Build history of the part. All positions in model axes, mm. Face numbers are marked on the shaded views. A direction names the side the tool comes from. Give positions to 0.01 mm unless a question says otherwise; leave off trailing zeros. Loops run counter-clockwise (first coordinate to the right, second up) from the corner with the lowest first, then second, coordinate; pieces in that order, holes last. Notation, with made-up numbers: (72, -26) -> (93, -26) arc R16 ccw to (93, -9) -> close; hole circle Ø4 at (18.25, 6). An arc over 180 degrees is marked (long way). Answer as a JSON object with one key per item and string values. Group by question number.
Q1. Band-saw the part on B-B, the plane x = 15. Write the cut outline in (y, z).
Q2. Tool access for the marked faces 4 and 5: list every direction of +Z, -Z, +X, -X, +Y, -Y with a clear straight run to the whole face (end or side of a thin tool).
Q3. Band-saw the part on A-A, the plane y = -3.75. Write the cut outline in (x, z).
Q4. Drop flat-ended pins along their axis: pin 1 (2 mm diameter, centred on y = -4, z = 7, fed in from +X); pin 2 (6 mm diameter, centred on x = 16.5, z = 12.5, fed in from -Y); pin 3 (2 mm diameter, centred on y = -3.5, z = 4.5, fed in from +X); pin 4 (2 mm diameter, centred on x = 13, y = -2.5, fed in from -Z). Give the stop position or say it passes through.
Q5. Band-saw the part on D-D, the plane z = 13.5. Write the cut outline in (x, y), plus the area to 3 significant figures.
Q6. Wall check: probe 1 along X at (y, z) = (-3.85, 11.75); probe 2 along X at (y, z) = (-1.45, 7.5); probe 3 along Z at (x, y) = (13.5, -1.4). Give the ranges that are in metal, low to high. Write a range as from..to.
Q7. Band-saw the part on C-C, the plane z = 7.5. Write the cut outline in (x, y).
Q8. Two-plate mould, pull along X, no slides. Class the marked faces 1, 2 and 3: pulls with the +X half, pulls with the -X half, needs draft (parallel to the pull), parting line crosses it, or undercut.
from build123d import *

# Parameters (mm, degrees)
BOSS_EXTRUDE1_DEPTH = 15
FILLET1_R           = 1
FILLET2_R           = 1
FILLET3_R           = 1
FILLET4_R           = 1
SKETCH2_R           = 2.25
CUT_EXTRUDE1_DEPTH  = 5


with BuildPart() as part:
    # Sketch1 → Boss-Extrude1 (new body)
    with BuildSketch(Plane.XY):
        Polygon((0, 0), (45, 0), (45, -2), (30, -2), (30, -5), (25, -5), (25, -2), (5, -2), (5, -5), (0, -5), align=None)
    extrude(amount=BOSS_EXTRUDE1_DEPTH)

    # Fillet1
    fillet1_edges = [part.edges().sort_by_distance(p)[0] for p in [
        (0, 0, 7.5),
    ]]
    fillet(fillet1_edges, radius=FILLET1_R)

    # Fillet2
    fillet2_edges = [part.edges().sort_by_distance(p)[0] for p in [
        (5, -2, 7.5),
    ]]
    fillet(fillet2_edges, radius=FILLET2_R)

    # Fillet3
    fillet3_edges = [part.edges().sort_by_distance(p)[0] for p in [
        (25, -2, 7.5),
    ]]
    fillet(fillet3_edges, radius=FILLET3_R)

    # Fillet4
    fillet4_edges = [part.edges().sort_by_distance(p)[0] for p in [
        (30, -2, 7.5),
    ]]
    fillet(fillet4_edges, radius=FILLET4_R)

    # Sketch2 → Cut-Extrude1 (cut)
    with BuildSketch(Plane(origin=(0, 0, 0), x_dir=(1, 0, 0), z_dir=(0, 1, 0))):
        with Locations(Location((15, -7.5, 0), (0, 0, 270))):
            Circle(SKETCH2_R)
    extrude(amount=-CUT_EXTRUDE1_DEPTH, mode=Mode.SUBTRACT)


solid = part.part
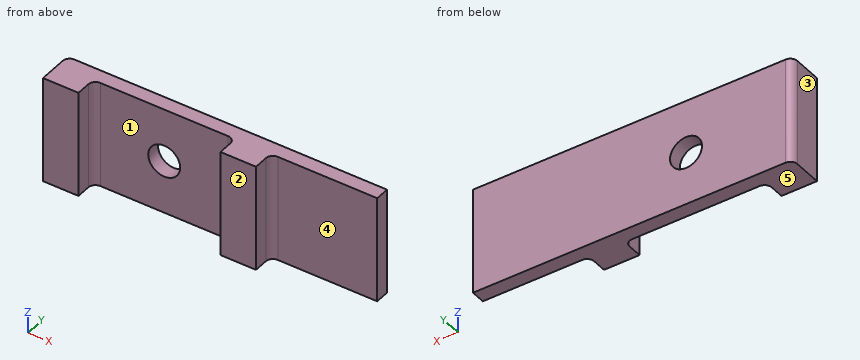
Worked answers:
{
 "1": {"outline": "(-2, 0) -> (0, 0) -> (0, 5.25) -> (-2, 5.25) -> close; (-2, 9.75) -> (0, 9.75) -> (0, 15) -> (-2, 15) -> close"},
 "2": {"face 4": "+Z, -Z, +X, -Y", "face 5": "-Z, +X, -X, +Y, -Y"},
 "3": {"outline": "(0, 0) -> (5, 0) -> (5, 15) -> (0, 15) -> close; (25, 0) -> (30, 0) -> (30, 15) -> (25, 15) -> close"},
 "4": {"pin 1": "x = 30", "pin 2": "y = -2", "pin 3": "x = 30.13", "pin 4": "z = 0"},
 "5": {"outline": "(0, -5) -> (5, -5) -> (5, -3) arc R1 cw to (6, -2) -> (24, -2) arc R1 cw to (25, -3) -> (25, -5) -> (30, -5) -> (30, -3) arc R1 cw to (31, -2) -> (45, -2) -> (45, 0) -> (1, 0) arc R1 ccw to (0, -1) -> close", "area": "120 mm2"},
 "6": {"probe 1": "0..5, 25..30", "probe 2": "0..12.75, 17.25..45", "probe 3": "0..5.82, 9.18..15"},
 "7": {"outline": "(0, -5) -> (5, -5) -> (5, -3) arc R1 cw to (6, -2) -> (12.75, -2) -> (12.75, 0) -> (1, 0) arc R1 ccw to (0, -1) -> close; (17.25, -2) -> (24, -2) arc R1 cw to (25, -3) -> (25, -5) -> (30, -5) -> (30, -3) arc R1 cw to (31, -2) -> (45, -2) -> (45, 0) -> (17.25, 0) -> close"},
 "8": {"face 1": "undercut", "face 2": "needs draft", "face 3": "pulls with the -X half"}
}
